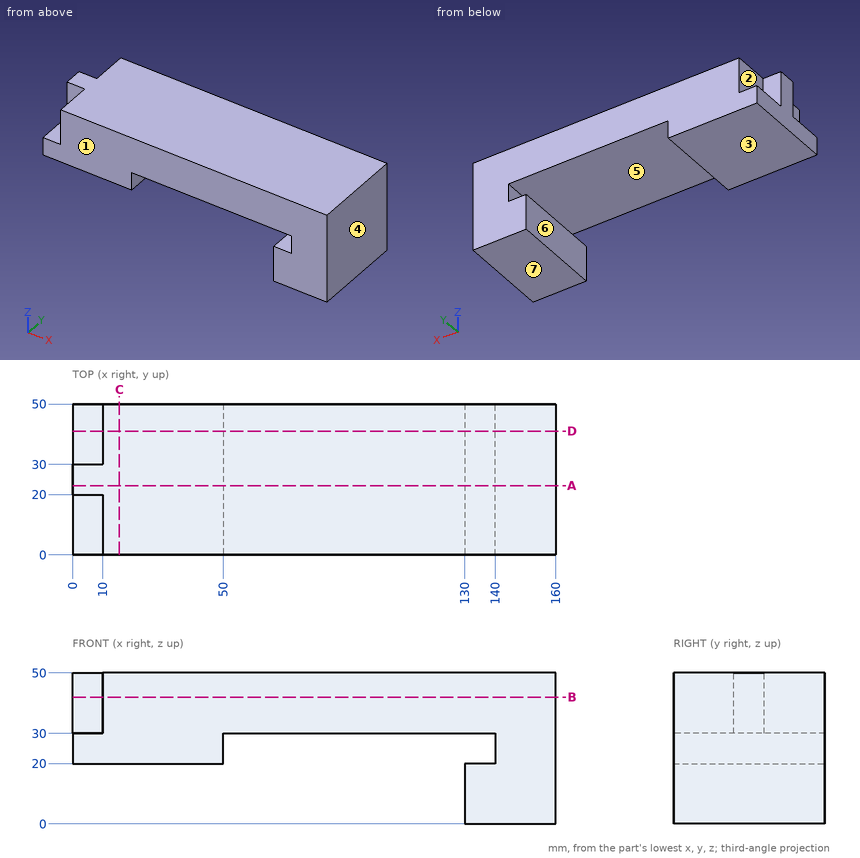
Could you check a few things on this drawing? It's one solid part, dimensions in mm from its lowest x, y, z. A direction names the side the tool comes from. Coordinates: 2 decimals unless noted, no trailing zeros. Write each loop counter-clockwise with the first axis right and the second up, starting at its lowest first coordinate (ties: lowest second). Pieces come first, ordered by that corner, then holes. Notation, with made-up numbers: (-2.5, 73.25) - (56.5, 73.25) arc R27 cw to (56.5, 89.25) - close; hole circle Ø5 at (83, 14.5). An arc over 180 degrees is marked (long way). Put each result on its own line as item: value. Start each with the question number.
Q1. Thinking about a two-plate mould opening in X: for the marked faces 4, 5, 6 and 7, which applies, pulls with the +X half, pulls with the -X half, needs draft (parallel to the pull), parting line crosses it, or undercut?
Q2. Please list where these lines run through material, in increasing order: L1, parallel to Z at x = 134.5, y = 28; L2, parallel to X at y = 43, z = 12; L3, parallel to X at y = 4, z = 28.
Q3. I want a section at C-C on x = 15.5. Write out the boundary of the cut face in (y, z), plus the area to 3 significant figures.
Q4. I want a section at B-B on z = 42. Write out the boundary of the cut face in (x, y), plus the area to 3 significant figures.
Q5. I want a section at D-D on y = 41. Write out the boundary of the cut face in (x, z).
Q6. I'm going to push flat-ended pins straight in: P1, Ø2, axis at x = 28, y = 35.5, coming from the -Z side; P2, Ø11, axis at x = 3.5, z = 41, coming from the +Y side; P3, Ø15, axis at x = 108, y = 21, coming from the -Z side; P4, Ø8, axis at x = 123, z = 25, coming from the +Y side. Where does each tip first touch, or does it pass through?
Q7. I want a section at A-A on y = 23. Write out the boundary of the cut face in (x, z), plus the area to 3 significant figures.
Q8. Which directions (+Z, -Z, +X, -X, +Y, -Y) give clear straight access to the entire face, cutting with the end or side of a thin tool? Please do the marked faces 1, 2 and 3.
Checks:
1. face 4: pulls with the +X half
1. face 5: undercut
1. face 6: pulls with the -X half
1. face 7: needs draft
2. L1: 0 to 20, 30 to 50
2. L2: 130 to 160
2. L3: 0 to 50, 140 to 160
3. outline: (0, 20) - (50, 20) - (50, 50) - (0, 50) - close
3. area: 1,500 mm²
4. outline: (0, 20) - (10, 20) - (10, 0) - (160, 0) - (160, 50) - (10, 50) - (10, 30) - (0, 30) - close
4. area: 7,600 mm²
5. outline: (0, 20) - (50, 20) - (50, 30) - (140, 30) - (140, 20) - (130, 20) - (130, 0) - (160, 0) - (160, 50) - (10, 50) - (10, 30) - (0, 30) - close
6. P1: z = 20
6. P2: y = 30
6. P3: z = 30
6. P4: through
7. outline: (0, 20) - (50, 20) - (50, 30) - (140, 30) - (140, 20) - (130, 20) - (130, 0) - (160, 0) - (160, 50) - (0, 50) - close
7. area: 4,500 mm²
8. face 1: +Z, -Z, +X, -X, -Y
8. face 2: +Z, -X, +Y
8. face 3: -Z, -X, +Y, -Y
